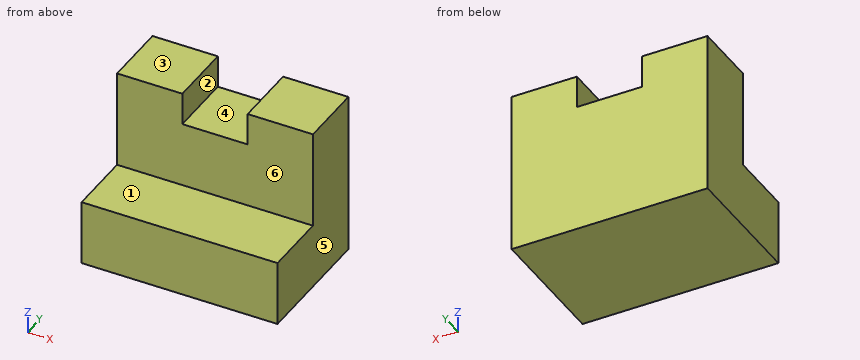
from build123d import *

# Parameters (mm, degrees)
F1_DEPTH = 38.1
F2_W     = 12.7
F2_H     = 6.35
F3_DEPTH = 12.7


with BuildPart() as f1:
    # F0 (on Right) → F1 (new body)
    with BuildSketch(Plane.YZ):
        Polygon((0, 0), (0, 31.75), (-12.7, 31.75), (-12.7, 12.7), (-25.4, 12.7), (-25.4, 0), align=None)
    extrude(amount=F1_DEPTH)

    # F2 (on Front) → F3 (cut)
    with BuildSketch(Plane.XZ):
        with Locations((19.05, 28.587072)):
            Rectangle(F2_W, F2_H)
    extrude(amount=F3_DEPTH, mode=Mode.SUBTRACT)


solid = f1.part
CAD build for the part. Positions are in the model's coordinates, mm. Face numbers are marked on the shaded views. A direction names the side the tool comes from. Coordinates: 2 decimals unless noted, no trailing zeros. Write each loop counter-clockwise with the first axis right and the second up, starting at its lowest first coordinate (ties: lowest second). Pieces come first, ordered by that corner, then holes. Notation, with made-up numbers: (43, 65.25) - (96, 65.25) arc R26 cw to (96, 104.25) - close; hole circle Ø10 at (-20.75, 83). An arc over 180 degrees is marked (long way). Use a Markdown table: item, result. Add a question column.
Item 1: Mould opens along X. For the marked faces 4, 5 and 6 say: pulls with the +X half, pulls with the -X half, needs draft (parallel to the pull), parting line crosses it, or undercut.
Item 2: 3-axis set-ups, long thin cutter, end or side, ignore diameter. For the marked faces 1, 2 and 3: which of +Z, -Z, +X, -X, +Y, -Y reach the whole face in a straight line?
Item 3: Band-saw the part on D-D, the plane x = 19. Give the cut face in (y, z).
Item 4: Band-saw the part on A-A, the plane x = 11.5. Give the cut face in (y, z).
Item 5: Drill centre lines: L1, parallel to Y at x = 4.5, z = 26; L2, parallel to X at y = -10.5, z = 26; L3, parallel to Z at x = 16, y = -4. Where is each one in solid material? Low to high. Write a range as from..to.
Item 6: Band-saw the part on B-B, the plane y = -6. Give the cut face in (x, z).
Item 7: Flat gauge pins, fed straight in: pin 1 (5 mm diameter, centred on x = 14.5, z = 15.5, fed in from -Y); pin 2 (6 mm diameter, centred on x = 28.5, y = -18.5, fed in from +Z); pin 3 (4 mm diameter, centred on x = 18, y = -5.5, fed in from +Z). Where does each tip first touch, or does it go through?
Item 8: Band-saw the part on C-C, the plane z = 18. Give the cut face in (x, y).
Numbers:
| question | item | result |
|---|---|---|
| 1 | face 4 | undercut |
| 1 | face 5 | pulls with the +X half |
| 1 | face 6 | needs draft |
| 2 | face 1 | +Z, +X, -X, -Y |
| 2 | face 2 | +Z, +Y, -Y |
| 2 | face 3 | +Z, +X, -X, +Y, -Y |
| 3 | outline | (-25.4, 0) - (0, 0) - (0, 25.41) - (-12.7, 25.41) - (-12.7, 12.7) - (-25.4, 12.7) - close |
| 4 | outline | (-25.4, 0) - (0, 0) - (0, 31.75) - (-12.7, 31.75) - (-12.7, 12.7) - (-25.4, 12.7) - close |
| 5 | L1 | -12.7..0 |
| 5 | L2 | 0..12.7, 25.4..38.1 |
| 5 | L3 | 0..25.41 |
| 6 | outline | (0, 0) - (38.1, 0) - (38.1, 31.75) - (25.4, 31.75) - (25.4, 25.41) - (12.7, 25.41) - (12.7, 31.75) - (0, 31.75) - close |
| 7 | pin 1 | y = -12.7 |
| 7 | pin 2 | z = 12.7 |
| 7 | pin 3 | z = 25.41 |
| 8 | outline | (0, -12.7) - (38.1, -12.7) - (38.1, 0) - (0, 0) - close |
